The drawing under review shows one solid part. Ordinate dimensions are in mm from its lowest x, y, z. A direction names the side the tool comes from. Coordinates: 2 decimals unless noted, no trailing zeros. Write each loop counter-clockwise with the first axis right and the second up, starting at its lowest first coordinate (ties: lowest second). Pieces come first, ordered by that corner, then holes.
Q1. Add section D-D, the plane x = 34. Give the boundary of the cut face in (y, z), plus the area to 3 significant figures.
Q2. Machinability: for the marked faces 1 and 2, which of the approach directions +Z, -Z, +X, -X, +Y, -Y give a long, thin tool a straight path to every point of the face, cutting with its end or side? Answer none if there is none.
Q3. Add section A-A, the plane y = 30. Give the boundary of the cut face in (x, z), plus the area to 3 significant figures.
Q4. To check wall thickness, follow probe 1 along Y at (x, z) = (19, 1.2); probe 2 along Y at (x, z) = (23.5, 3.5); probe 3 along X at (y, z) = (0.6, 29). State the ranges of each line that lie inside material, in increasing order.
Q5. Clearance check with flat-ended pins moving along their axes: pin 1 Ø2 at (x, y) = (19.5, 12) entering from +Z; pin 2 Ø8 at (x, z) = (19, 11) entering from +Y; pin 3 Ø1 at (x, y) = (19, 4.5) entering from +Z. State where each tip first meets the part, or that it passes through.
Q6. Add section C-C, the plane x = 19. Give the boundary of the cut face in (y, z).
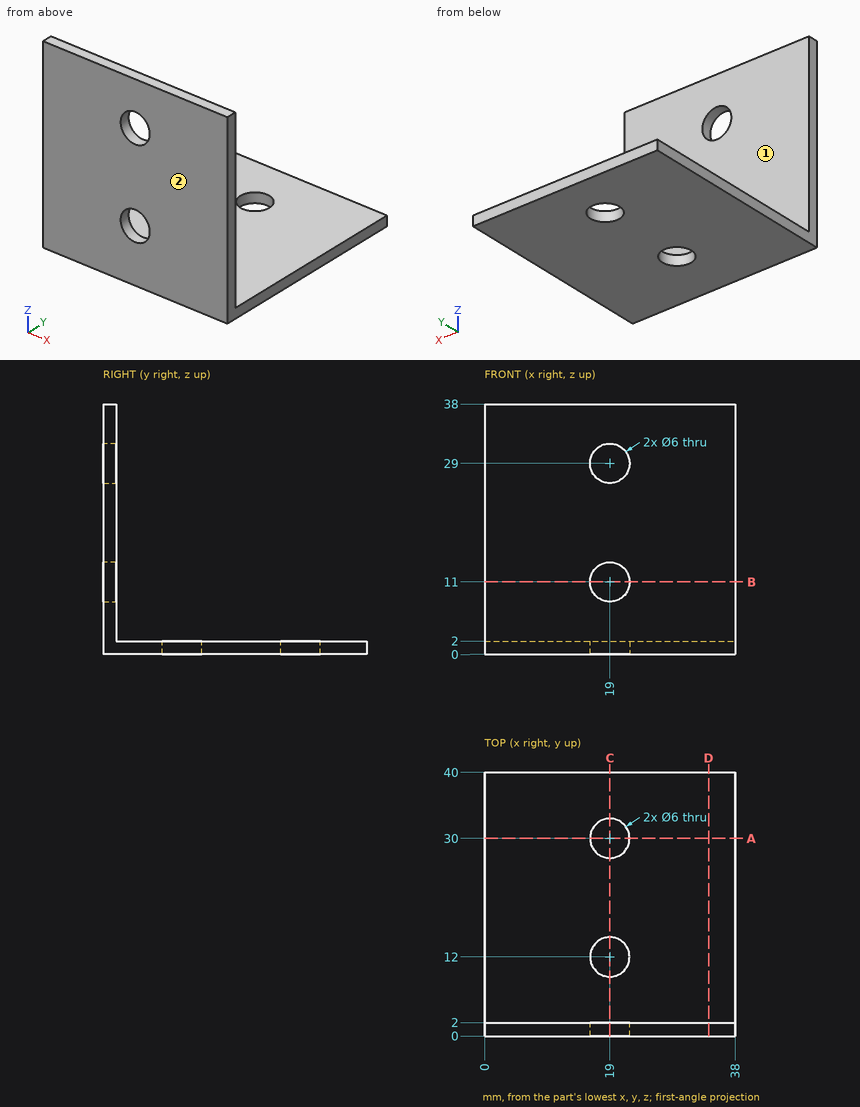
Here are the results:
1. outline: (0, 0) - (40, 0) - (40, 2) - (2, 2) - (2, 38) - (0, 38) - close
1. area: 152 mm2
2. face 1: +Z, +X, -X, +Y
2. face 2: +Z, -Z, +X, -X, -Y
3. outline: (0, 0) - (16, 0) - (16, 2) - (0, 2) - close; (22, 0) - (38, 0) - (38, 2) - (22, 2) - close
3. area: 64.0 mm2
4. probe 1: y = 0 to 9, 15 to 27, 33 to 40
4. probe 2: y = 0 to 2
4. probe 3: x = 0 to 16, 22 to 38
5. pin 1: passes through
5. pin 2: stops at y = 2
5. pin 3: stops at z = 2
6. outline: (0, 0) - (9, 0) - (9, 2) - (2, 2) - (2, 8) - (0, 8) - close; (0, 14) - (2, 14) - (2, 26) - (0, 26) - close; (0, 32) - (2, 32) - (2, 38) - (0, 38) - close; (15, 0) - (27, 0) - (27, 2) - (15, 2) - close; (33, 0) - (40, 0) - (40, 2) - (33, 2) - close
